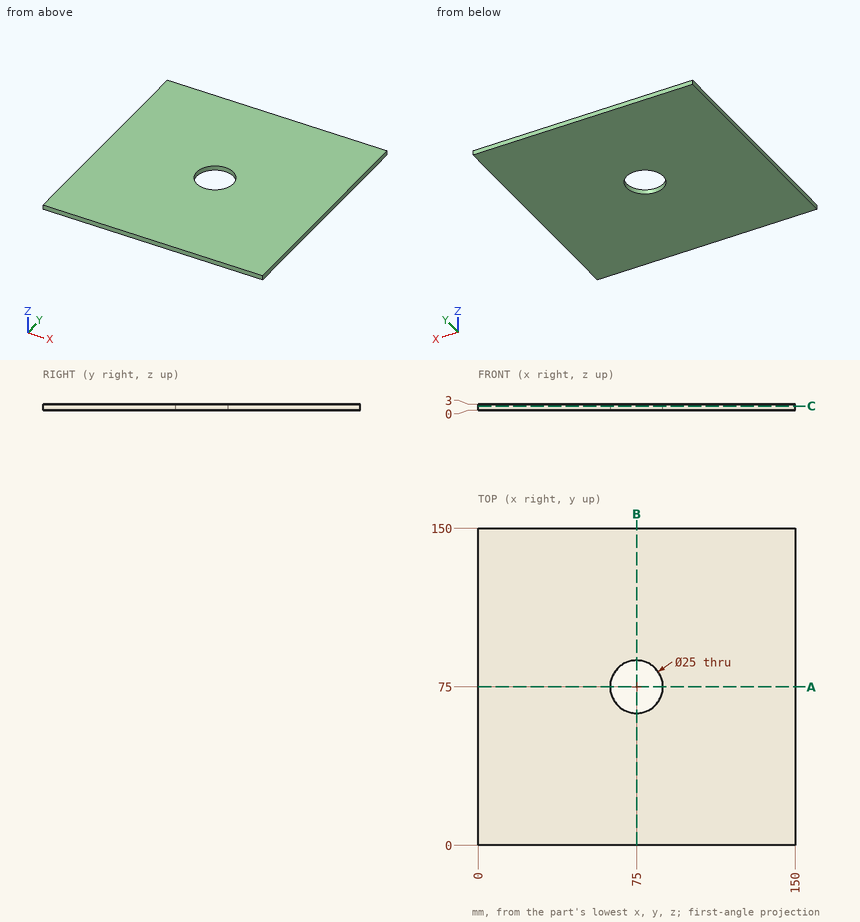
Can you work these out from the drawing? Everything is in mm from the part's minimum corner. Coordinates: 2 decimals unless noted, no trailing zeros. Write each loop counter-clockwise with the first axis right and the second up, starting at its lowest first coordinate (ties: lowest second). Pieces come first, ordered by that corner, then holes. Notation, with made-up numbers: (6.5, 62.5) -> (44.5, 62.5) arc R22 ccw to (44.5, 70.5) -> close; hole circle Ø10 at (25, 13.5). An arc over 180 degrees is marked (long way). Return JSON: item names as keys, results as strings.
(1) I need wall thicknesses on L1, parallel to Y at x = 75, z = 1; L2, parallel to X at y = 81.5, z = 0.2; L3, parallel to X at y = 73, z = 2.6. Which ranges of each line are inside material? Lowest first, please.
Numbers:
{"L1": "y = 0 to 62.5, 87.5 to 150", "L2": "x = 0 to 64.32, 85.68 to 150", "L3": "x = 0 to 62.66, 87.34 to 150"}
(2) Imagine slicing it at A-A, the plane y = 75. Please give me the cut outline in (x, z).
Numbers:
{"outline": "(0, 0) -> (62.5, 0) -> (62.5, 3) -> (0, 3) -> close; (87.5, 0) -> (150, 0) -> (150, 3) -> (87.5, 3) -> close"}
(3) Imagine slicing it at C-C, the plane z = 2.05. Please give me the cut outline in (x, y).
Numbers:
{"outline": "(0, 0) -> (150, 0) -> (150, 150) -> (0, 150) -> close; hole circle Ø25 at (75, 75)"}
(4) I'm going to push a flat-ended pin straight in: pin 1 (2 mm diameter, centred on x = 119, y = 21, fed in from -Z). Where does the tip first touch, or does it pass through?
Numbers:
{"pin 1": "stops at z = 0"}
